```python
from build123d import *

# Parameters (mm, degrees)
SKETCH1_R           = 4
BOSS_EXTRUDE1_DEPTH = 70
SKETCH2_W           = 4.7
SKETCH2_H           = 5.4
BOSS_EXTRUDE4_DEPTH = 30


with BuildPart() as part:
    # Sketch1 → Boss-Extrude1 (new body)
    with BuildSketch(Plane.XY):
        Circle(SKETCH1_R)
    extrude(amount=BOSS_EXTRUDE1_DEPTH)

    # Sketch2 → Boss-Extrude4 (add)
    with BuildSketch(Plane.XY.offset(70)):
        with Locations((0, 4)):
            Rectangle(SKETCH2_W, SKETCH2_H)
    extrude(amount=-BOSS_EXTRUDE4_DEPTH)


solid = part.part
```
Geometry: final body of the model. Coordinates: model frame, mm. A direction names the side the tool comes from. Round coordinates to 2 decimals unless told otherwise and drop trailing zeros. Order: outer loops, then holes, each group sorted by start corner. A loop starts at its lowest first (then second) coordinate and runs counter-clockwise, first axis right, second up. Notation, with made-up numbers: (20, 75) -> (42, 75) arc R12 ccw to (42, 94) -> close; hole circle Ø5 at (40, 44.25). An arc over 180 degrees is marked (long way). Use one line per item in the form item = value. Start each with the question number.
1. Cut plane A-A (x = 0). Return the cut outline in (y, z).
2. Cut plane D-D (z = 30.5). Return the cut outline in (x, y).
3. Cut plane B-B (z = 45.5). Return the cut outline in (x, y).
4. Pin query (flat end, axial travel): pin 1 Ø2 at (y, z) = (3, 16.5) entering from +X; pin 2 Ø4 at (y, z) = (4, 24) entering from -X; pin 3 Ø3 at (y, z) = (5, 49.5) entering from -X; pin 4 Ø4 at (x, y) = (1, 5.5) entering from -Z. Return the tip coordinate at first contact, or that it passes through.
5. Reachability of faces 1 (the face through (-0.867, -3.905, 34.51)), 2 (the face through (0, 0, 0)), 3 (the face through (-2.35, 5, 55)), 4 (the face through (2.35, 5, 55)) from +Z, -Z, +X, -X, +Y, -Y: full face, straight path, thin tool, end or side. Return the list, or none.
6. Cut plane C-C (y = 5.75). Return the cut outline in (x, z), then the cut area to 3 significant figures.
7. Line query: probe 1 along X at (y, z) = (5.5, 66); probe 2 along Y at (x, z) = (0.25, 67); probe 3 along X at (y, z) = (0.25, 8.5). Output: solid intervals per line, ascending.
Solution:
q1.outline = (-4, 0) -> (4, 0) -> (4, 40) -> (6.7, 40) -> (6.7, 70) -> (-4, 70) -> close
q2.outline = circle Ø8 at (0, 0)
q3.outline = (-2.35, 3.24) arc R4 ccw (long way) to (2.35, 3.24) -> (2.35, 6.7) -> (-2.35, 6.7) -> close
q4.pin_1 = 3.46
q4.pin_2 = -3.46
q4.pin_3 = -2.35
q4.pin_4 = 0
q5.face_1 = -Z
q5.face_2 = -Z, +X, -X, +Y, -Y
q5.face_3 = +Z, -Z, -X, +Y
q5.face_4 = +Z, -Z, +X, +Y
q6.outline = (-2.35, 40) -> (2.35, 40) -> (2.35, 70) -> (-2.35, 70) -> close
q6.area = 141 mm^2
q7.probe_1 = -2.35 to 2.35
q7.probe_2 = -3.99 to 6.7
q7.probe_3 = -3.99 to 3.99
